The model under review builds one solid part; all positions refer to its coordinate system, in mm. Face numbers are marked on the shaded views. Coordinates: 2 decimals unless noted, no trailing zeros.
```python
from build123d import *

# Parameters (mm, degrees)
F3_DEPTH = 52.81897
F4_R     = 10


with BuildPart() as f1:
    # F0 (on Front) → F1 (revolve)
    with BuildSketch(Plane.XZ):
        with BuildLine():
            Line((0, 10), (0, 0))
            Line((0, 0), (26.5, 0))
            Line((26.5, 0), (26.5, 55))
            Line((26.5, 55), (25.092501, 55))
            ThreePointArc((25.092501, 55), (23.849016, 54.566444), (23.144652, 53.453747))
            ThreePointArc((23.144652, 53.453747), (17.005279, 31.423188), (9, 10))
            Line((9, 10), (0, 10))
        make_face()
    revolve(axis=Axis((0, 0, 17.288097), (0, 0, 1)))

    # F2 (on Right) → F3 (cut, symmetric)
    with BuildSketch(Plane.YZ):
        with BuildLine():
            ThreePointArc((-4.980726, 55), (144.261109, 36.559124), (224.721762, 163.59957))
            ThreePointArc((224.721762, 163.59957), (24.13583, 290.640016), (-4.980726, 55))
        make_face()
    extrude(amount=F3_DEPTH, both=True, mode=Mode.SUBTRACT)

    # F4
    f4_edges = [f1.edges().sort_by_distance(p)[0] for p in [
        (-9, 0, 10),
    ]]
    fillet(f4_edges, radius=F4_R)


solid = f1.part
```
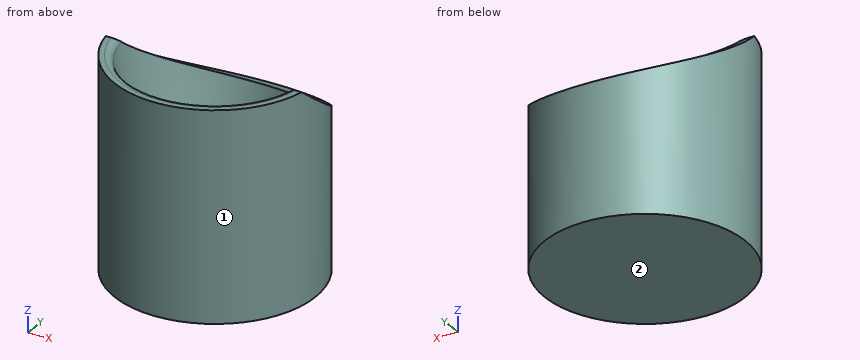
(1) For pin 1 Ø1 at (x, z) = (3, 34) entering from -Y; pin 2 Ø10 at (x, z) = (-15.5, 23) entering from +Y; pin 3 Ø8 at (x, y) = (-7.5, -9.5) entering from -Z; pin 4 Ø3 at (x, z) = (-9.5, 5.5) entering from +Y, all flat-tipped, find the tip position at first contact; note any pin that passes through.
A:
pin 1: stops at y = -26.38
pin 2: stops at y = 24.33
pin 3: stops at z = 0
pin 4: stops at y = 25.26
(2) Draft analysis for pull direction Z (two halves, no side actions). For the marked faces 1 and 2, state which applies: released by +Z, released by -Z, zero draft, split by the parting line, or undercut.
A:
face 1: zero draft
face 2: released by -Z
(3) Wall thickness on probe 1 along Y at (x, z) = (11, 27); probe 2 along X at (y, z) = (-10, 16.5); probe 3 along Y at (x, z) = (-12.5, 23): over which ranges is each line inside the solid? List them lowest first.
A:
probe 1: y = -24.11 to -10.95, 10.95 to 24.11
probe 2: x = -24.54 to -5.98, 5.98 to 24.54
probe 3: y = -23.37 to -6.54, 6.54 to 23.37
